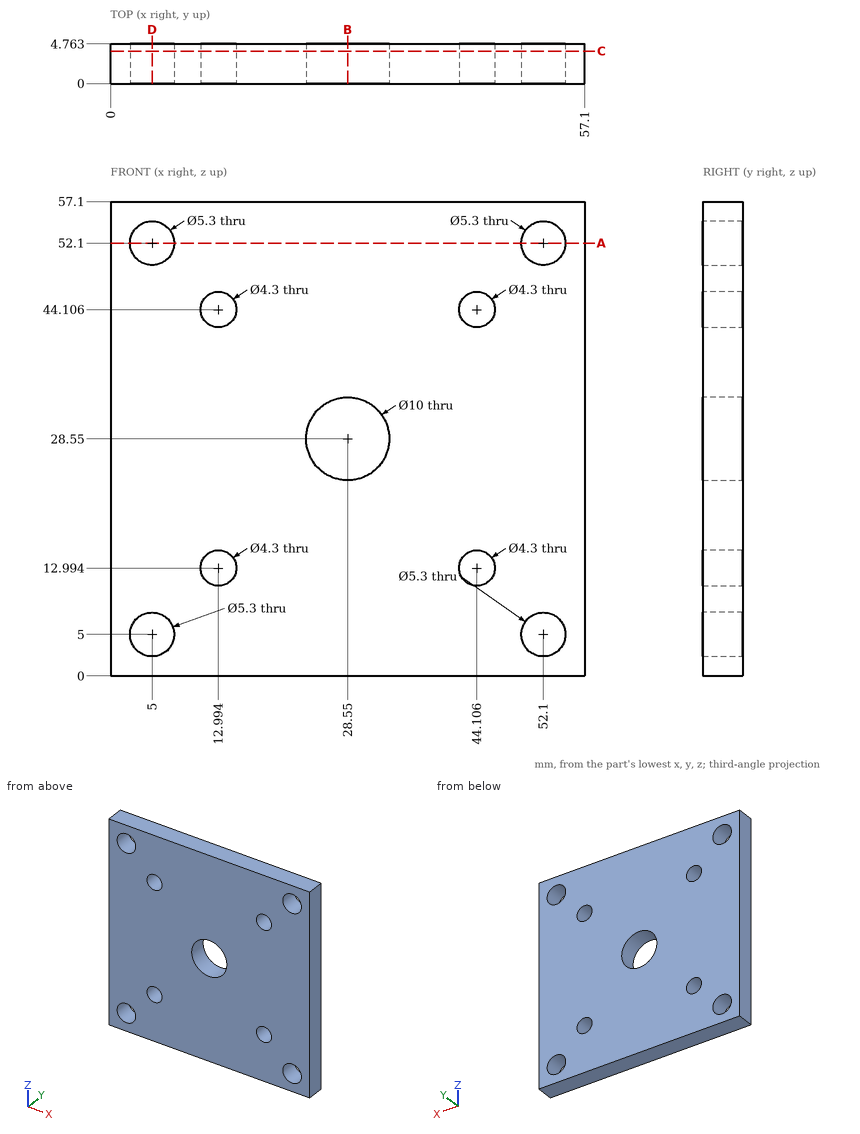
Design review of the part shown in the three views and the two pictorial views. Dimensions are in mm from the part's minimum x, y and z. Give positions to 0.01 mm unless a question says otherwise; leave off trailing zeros. Order: outer loops, then holes, each group sorted by start corner. A loop starts at its lowest first (then second) coordinate and runs counter-clockwise, first axis right, second up. Notation, with made-up numbers: M 36,63 L 84,63 A16 ccw 84,68 Z; hole C 83.5,-27.5 d8. An arc over 180 degrees is marked long. Answer in a Markdown table with one row per item. Add a question column.
(1) Consider section A-A on z = 52.1. State the section outline as (x, y) points.
(2) For pin 1 (3 mm diameter, centred on x = 5, z = 52.1, fed in from +Y); pin 2 (3 mm diameter, centred on x = 23, z = 13, fed in from -Y), all flat-tipped, find the tip position at first contact; note any pin that passes through.
(3) Consider section C-C on y = 3.9. Give the number of separate pieces and of enclosed holes in the cut face, and give its area (3 significant figures).
(4) Consider section B-B on x = 28.55. State the section outline as (y, z) points, and give its area (3 significant figures).
(5) Consider section D-D on x = 5. State the section outline as (y, z) points.
(6) Wall thickness on probe 1 along X at (y, z) = (3.45, 52.1); probe 2 along X at (y, z) = (3.1, 44); probe 3 along Z at (x, y) = (14, 3.35) (1 decimal): over which ranges is each line inside the solid? List them lowest first. Write a range as [from, to].
Evaluation:
| question | item | result |
|---|---|---|
| 1 | outline | M 0,0 L 2.35,0 L 2.35,4.76 L 0,4.76 Z; M 7.65,0 L 49.45,0 L 49.45,4.76 L 7.65,4.76 Z; M 54.75,0 L 57.1,0 L 57.1,4.76 L 54.75,4.76 Z |
| 2 | pin 1 | passes through |
| 2 | pin 2 | stops at y = 0 |
| 3 | separate pieces | 1 |
| 3 | enclosed holes | 9 |
| 3 | area | 3,040 mm^2 |
| 4 | outline | M 0,0 L 4.76,0 L 4.76,23.55 L 0,23.55 Z; M 0,33.55 L 4.76,33.55 L 4.76,57.1 L 0,57.1 Z |
| 4 | area | 224 mm^2 |
| 5 | outline | M 0,0 L 4.76,0 L 4.76,2.35 L 0,2.35 Z; M 0,7.65 L 4.76,7.65 L 4.76,49.45 L 0,49.45 Z; M 0,54.75 L 4.76,54.75 L 4.76,57.1 L 0,57.1 Z |
| 6 | probe 1 | x = [0, 2.35], [7.65, 49.45], [54.75, 57.1] |
| 6 | probe 2 | x = [0, 10.85], [15.14, 41.96], [46.25, 57.1] |
| 6 | probe 3 | z = [0, 11.1], [14.9, 42.2], [46, 57.1] |
